Build history of the part. All positions in model axes, mm. A direction names the side the tool comes from. Give positions to 0.01 mm unless a question says otherwise; leave off trailing zeros. Write each loop counter-clockwise with the first axis right and the second up, starting at its lowest first coordinate (ties: lowest second). Pieces come first, ordered by that corner, then holes. Notation, with made-up numbers: M 85.5,26.5 L 104.5,26.5 A20 cw 104.5,60.5 Z; hole C 35.25,-22.75 d9. An arc over 180 degrees is marked long. Return JSON: item names as keys, results as strings. Group by question number.
Q1. Pull direction Y, two halves, no side cores. Call faces 1 (the cylindrical face through (75.6, 98.1, 113.8)), 2 (the flat face through (50, 3, 102.544)), 3 (the flat face through (-38, 6.35, -41)): +Y half, -Y half, draft (parallel to the pull), parting line (faces both ways), or undercut.
Q2. Band-saw the part on B-B, the plane z = 119. Give the cut face in (x, y).
Q3. Band-saw the part on C-C, the plane x = -3. Give the cut face in (y, z) (3 decimals), then the cut area to 3 significant figures.
Q4. Flat gauge pins, fed straight in: pin 1 Ø4 at (y, z) = (68.5, -58) entering from -X; pin 2 Ø2.5 at (x, z) = (13.5, -44.5) entering from +Y; pin 3 Ø4 at (y, z) = (65.5, -57.5) entering from +X. Where does each tip first touch, or does it go through?
Q5. Band-saw the part on A-A, the plane x = -42. Give the cut face in (y, z).
Q6. Wall check: probe 1 along Z at (x, y) = (36.5, 7); probe 2 along X at (y, z) = (79, 106); probe 3 along X at (y, z) = (116, 84.5). Give the ranges that are in metal, low to high.
Q7. Tool access for faces 4 (the cylindrical face through (73.5, 72.3, 111.4)), 5 (the flat face through (-63.484, 71.623, 112.024)), 6 (the flat face through (-19.347, 29, -50)): list every direction of +Z, -Z, +X, -X, +Y, -Y with a clear straight run to the whole face (end or side of a thin tool).
Q8. Band-saw the part on D-D, the plane y = 103. Give the cut face in (x, z), then the cut area to 3 significant figures.
from build123d import *

# Parameters (mm, degrees)
BOSS_EXTRUDE1_DEPTH = 6.35
BOSS_EXTRUDE2_DEPTH = 114.3
SKETCH3_W           = 69.2
SKETCH3_H           = 50
CUT_EXTRUDE1_DEPTH  = 31.71
FILLET1_R           = 2.54
CUT_EXTRUDE2_DEPTH  = 3.175
FILLET2_R           = 2.54
SKETCH8_W           = 50.8
SKETCH8_H           = 6.35
BOSS_EXTRUDE3_DEPTH = 12.7
SKETCH9_W           = 27.302002056
SKETCH9_H           = 3.175
BOSS_EXTRUDE4_DEPTH = 6.35
FILLET4_R           = 2.54
FILLET5_R           = 2.54


with BuildPart() as part:
    # Sketch1 → Boss-Extrude1 (new body)
    with BuildSketch(Plane(origin=(0, 0, 0), x_dir=(1, 0, 0), z_dir=(0, 1, 0))):
        with BuildLine():
            Line((-51.097477477, 62.55608588), (63.202522523, 62.55608588))
            ThreePointArc((63.202522523, 62.55608588), (72.182778644, 58.836342002), (75.902522523, 49.85608588))
            Line((75.902522523, 49.85608588), (75.902522523, -127.94391412))
            ThreePointArc((75.902522523, -127.94391412), (72.182778644, -136.924170241), (63.202522523, -140.64391412))
            Line((63.202522523, -140.64391412), (-51.097477477, -140.64391412))
            ThreePointArc((-51.097477477, -140.64391412), (-60.077733599, -136.924170241), (-63.797477477, -127.94391412))
            Line((-63.797477477, -127.94391412), (-63.797477477, 49.85608588))
            ThreePointArc((-63.797477477, 49.85608588), (-60.077733599, 58.836342002), (-51.097477477, 62.55608588))
        make_face()
        Polygon((-57.447477477, 24.45608588), (-57.447477477, -102.54391412), (-19.347477477, -102.54391412), (-19.347477477, -134.29391412), (31.452522523, -134.29391412), (31.452522523, -102.54391412), (69.552522523, -102.54391412), (69.552522523, 24.45608588), (31.452522523, 24.45608588), (31.452522523, 56.20608588), (-19.347477477, 56.20608588), (-19.347477477, 24.45608588), align=None, mode=Mode.SUBTRACT)
    extrude(amount=BOSS_EXTRUDE1_DEPTH)

    # Sketch2 → Boss-Extrude2 (add)
    with BuildSketch(Plane(origin=(0, 6.35, 0), x_dir=(1, 0, 0), z_dir=(0, 1, 0))):
        with BuildLine():
            Line((75.902522523, -127.94391412), (75.902522523, 49.85608588))
            ThreePointArc((75.902522523, 49.85608588), (72.182778644, 58.836342002), (63.202522523, 62.55608588))
            Line((63.202522523, 62.55608588), (-51.097477477, 62.55608588))
            ThreePointArc((-51.097477477, 62.55608588), (-60.077733599, 58.836342002), (-63.797477477, 49.85608588))
            Line((-63.797477477, 49.85608588), (-63.797477477, -127.94391412))
            ThreePointArc((-63.797477477, -127.94391412), (-60.077733599, -136.924170241), (-51.097477477, -140.64391412))
            Line((-51.097477477, -140.64391412), (63.202522523, -140.64391412))
            ThreePointArc((63.202522523, -140.64391412), (72.182778644, -136.924170241), (75.902522523, -127.94391412))
        make_face()
        with BuildLine():
            Line((69.552522523, -127.94391412), (69.552522523, 49.85608588))
            ThreePointArc((69.552522523, 49.85608588), (67.692650583, 54.346213941), (63.202522523, 56.20608588))
            Line((63.202522523, 56.20608588), (-51.097477477, 56.20608588))
            ThreePointArc((-51.097477477, 56.20608588), (-55.587605538, 54.346213941), (-57.447477477, 49.85608588))
            Line((-57.447477477, 49.85608588), (-57.447477477, -127.94391412))
            ThreePointArc((-57.447477477, -127.94391412), (-55.587605538, -132.43404218), (-51.097477477, -134.29391412))
            Line((-51.097477477, -134.29391412), (63.202522523, -134.29391412))
            ThreePointArc((63.202522523, -134.29391412), (67.692650583, -132.43404218), (69.552522523, -127.94391412))
        make_face(mode=Mode.SUBTRACT)
    extrude(amount=BOSS_EXTRUDE2_DEPTH)

    # Sketch3 → Cut-Extrude1 (cut)
    with BuildSketch(Plane(origin=(0, 0, -62.55608588), x_dir=(-1, 0, 0), z_dir=(0, 0, -1))):
        with Locations((-6.052522523, 60.325)):
            Rectangle(SKETCH3_W, SKETCH3_H)
    extrude(amount=-CUT_EXTRUDE1_DEPTH, mode=Mode.SUBTRACT)

    # Fillet1
    fillet1_edges = [part.edges().sort_by_distance(p)[0] for p in [
        (6.052522523, 85.325, -62.55608588),
        (-28.547477477, 60.325, -62.55608588),
        (40.652522523, 60.325, -62.55608588),
        (6.052522523, 35.325, -62.55608588),
    ]]
    fillet(fillet1_edges, radius=FILLET1_R)

    # Sketch6 → Cut-Extrude2 (cut)
    with BuildSketch(Plane.ZY.offset(63.797477477)):
        with BuildLine():
            Line((-49.85608588, 23.368), (103.519740541, 45.45891847))
            ThreePointArc((103.519740541, 45.45891847), (107.09072322, 47.24008694), (108.89391412, 50.8))
            Line((108.89391412, 50.8), (115.24391412, 93.037110429))
            ThreePointArc((115.24391412, 93.037110429), (113.736824756, 98.170115624), (108.842546446, 100.33))
            Line((108.842546446, 100.33), (-49.85608588, 97.282))
            Line((-49.85608588, 97.282), (-49.85608588, 23.368))
        make_face()
    cut_extrude2 = extrude(amount=-CUT_EXTRUDE2_DEPTH, mode=Mode.SUBTRACT)

    # Fillet2
    fillet2_edges = [part.edges().sort_by_distance(p)[0] for p in [
        (-60.622477477, 98.170115624, 113.736824756),
        (-60.622477477, 71.918555214, 112.06891412),
        (-60.622477477, 47.24008694, 107.09072322),
        (-60.622477477, 34.413459235, 26.83182733),
        (-60.622477477, 60.325, -49.85608588),
        (-60.622477477, 98.806, 29.493230283),
    ]]
    fillet(fillet2_edges, radius=FILLET2_R)

    # Sketch8 → Boss-Extrude3 (add)
    with BuildSketch(Plane.XY.offset(-56.20608588)):
        with Locations((6.052522523, 28.975)):
            Rectangle(SKETCH8_W, SKETCH8_H)
    extrude(amount=BOSS_EXTRUDE3_DEPTH)

    # Sketch9 → Boss-Extrude4 (add)
    with BuildSketch(Plane(origin=(0, 32.15, 0), x_dir=(1, 0, 0), z_dir=(0, 1, 0))):
        with Locations((17.801521495, 45.09358588)):
            Rectangle(SKETCH9_W, SKETCH9_H)
    extrude(amount=BOSS_EXTRUDE4_DEPTH)

    # Fillet4
    fillet4_edges = [part.edges().sort_by_distance(p)[0] for p in [
        (6.052522523, 25.8, -56.20608588),
    ]]
    fillet(fillet4_edges, radius=FILLET4_R)

    # Mirror2: Cut-Extrude2 across plane
    add(cut_extrude2.mirror(Plane(origin=(6.052522523, 0, 0), x_dir=(0, 0, 1), z_dir=(1, 0, 0))), mode=Mode.SUBTRACT)

    # Fillet5
    fillet5_edges = [part.edges().sort_by_distance(p)[0] for p in [
        (72.727522523, 98.170115624, 113.736824756),
        (72.727522523, 98.806, 29.493230283),
        (72.727522523, 34.413459235, 26.83182733),
        (72.727522523, 47.24008694, 107.09072322),
        (72.727522523, 71.918555214, 112.06891412),
    ]]
    fillet(fillet5_edges, radius=FILLET5_R)


solid = part.part
From the geometry:
{
 "1": {"face 1": "undercut", "face 2": "draft", "face 3": "+Y half"},
 "2": {"outline": "M -63.8,0 L -19.35,0 L -19.35,6.35 L -57.45,6.35 L -57.45,120.65 L -63.8,120.65 Z; M 31.45,0 L 75.9,0 L 75.9,120.65 L 69.55,120.65 L 69.55,6.35 L 31.45,6.35 Z"},
 "3": {"outline": "M 0,-62.556 L 32.785,-62.556 A2.54 ccw 35.325,-60.016 L 35.325,-56.206 L 32.15,-56.206 L 32.15,-43.506 L 25.8,-43.506 L 25.8,-53.666 A2.54 cw 23.26,-56.206 L 0,-56.206 Z; M 0,134.294 L 120.65,134.294 L 120.65,140.644 L 0,140.644 Z; M 85.325,-60.016 A2.54 ccw 87.865,-62.556 L 120.65,-62.556 L 120.65,-56.206 L 85.325,-56.206 Z", "area": "1,290 mm^2"},
 "4": {"pin 1": "stops at x = -62.21", "pin 2": "stops at y = 38.5", "pin 3": "stops at x = 74.58"},
 "5": {"outline": "M 0,-62.56 L 120.65,-62.56 L 120.65,-56.21 L 6.35,-56.21 L 6.35,-24.46 L 0,-24.46 Z; M 0,102.54 L 6.35,102.54 L 6.35,134.29 L 120.65,134.29 L 120.65,140.64 L 0,140.64 Z"},
 "6": {"probe 1": "z = -62.56 to -56.21, 134.29 to 140.64", "probe 2": "x = -60.62 to -57.45, 69.55 to 72.73", "probe 3": "x = -63.8 to -57.45, 69.55 to 75.9"},
 "7": {"face 4": "+X", "face 5": "-X", "face 6": "+Y"},
 "8": {"outline": "M -63.8,-49.86 A12.7 ccw -51.1,-62.56 L 63.2,-62.56 A12.7 ccw 75.9,-49.86 L 75.9,127.94 A12.7 ccw 63.2,140.64 L -51.1,140.64 A12.7 ccw -63.8,127.94 Z; hole M -57.45,-49.86 A6.35 ccw -51.1,-56.21 L 63.2,-56.21 A6.35 ccw 69.55,-49.86 L 69.55,127.94 A6.35 ccw 63.2,134.29 L -51.1,134.29 A6.35 ccw -57.45,127.94 Z", "area": "4,090 mm^2"}
}
